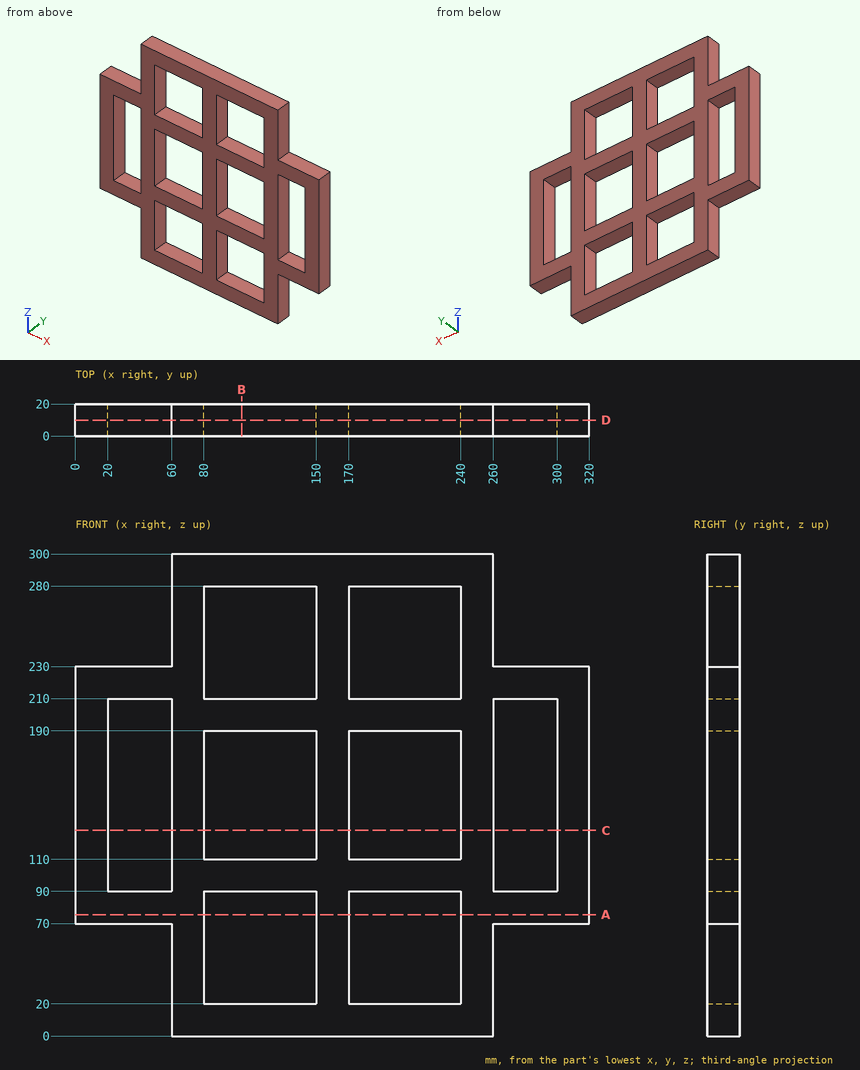
Geometry check sheet. Reference: drawing and pictorial views, mm from the part's lowest x, y, z. Coordinates: 2 decimals unless noted, no trailing zeros. Loops run counter-clockwise (first coordinate to the right, second up) from the corner with the lowest first, then second, coordinate; pieces in that order, holes last.
1) Sectioned sample at D-D (y = 10). Count the separate pieces of the cut face and the enclosed holes in it, and give its area (3 significant figures).
2) Sectioned sample at C-C (z = 128). Record the boundary of the cut face in (x, y).
3) Sectioned sample at B-B (x = 103.5). Record the boundary of the cut face in (y, z).
4) Material ranges on probe 1 along X at (y, z) = (15.75, 64); probe 2 along X at (y, z) = (14.75, 90.5); probe 3 along Z at (x, y) = (227.5, 8.75), recorded low to high.
5) Gauge pin test, flat ends, axial feed: pin 1 (6 mm diameter, centred on x = 299, y = 9, fed in from -Z); pin 2 (3 mm diameter, centred on x = 39.5, z = 225.5, fed in from -Y); pin 3 (6 mm diameter, centred on y = 7.5, z = 249, fed in from -X); pin 4 (6 mm diameter, centred on x = 49.5, y = 10.5, fed in from +Z). Record the tip position at first contact, or that the pin passes through.
6) Sectioned sample at A-A (z = 75.5). Record the boundary of the cut face in (x, y).
Check sheet entries:
1. separate pieces: 1
1. enclosed holes: 8
1. area: 38,800 mm2
2. outline: (0, 0) - (20, 0) - (20, 20) - (0, 20) - close; (60, 0) - (80, 0) - (80, 20) - (60, 20) - close; (150, 0) - (170, 0) - (170, 20) - (150, 20) - close; (240, 0) - (260, 0) - (260, 20) - (240, 20) - close; (300, 0) - (320, 0) - (320, 20) - (300, 20) - close
3. outline: (0, 0) - (20, 0) - (20, 20) - (0, 20) - close; (0, 90) - (20, 90) - (20, 110) - (0, 110) - close; (0, 190) - (20, 190) - (20, 210) - (0, 210) - close; (0, 280) - (20, 280) - (20, 300) - (0, 300) - close
4. probe 1: x = 60 to 80, 150 to 170, 240 to 260
4. probe 2: x = 0 to 20, 60 to 260, 300 to 320
4. probe 3: z = 0 to 20, 90 to 110, 190 to 210, 280 to 300
5. pin 1: stops at z = 70
5. pin 2: stops at y = 0
5. pin 3: stops at x = 60
5. pin 4: stops at z = 230
6. outline: (0, 0) - (80, 0) - (80, 20) - (0, 20) - close; (150, 0) - (170, 0) - (170, 20) - (150, 20) - close; (240, 0) - (320, 0) - (320, 20) - (240, 20) - close
